Verification items for the finished model (mm, model axes). Round coordinates to 2 decimals unless told otherwise and drop trailing zeros. Write each loop counter-clockwise with the first axis right and the second up, starting at its lowest first coordinate (ties: lowest second). Pieces come first, ordered by that corner, then holes. Notation, with made-up numbers: (-21, -2.75) -> (4, -2.75) arc R17 ccw to (4, 15.25) -> close; hole circle Ø5 at (-1.75, -4). An arc over 180 degrees is marked (long way). Answer as a JSON object with one key per item and string values. Group by question number.
(1) Scan lines: L1, parallel to Y at x = 0, z = 1.7; L2, parallel to Y at x = 123, z = 3.9; L3, parallel to Y at x = 27, z = 0.3. Record each from-to range of solid material in increasing order. Write a range as from..to.
(2) Draft check along X on faces 1 (the face through (5.76, 1, 2.46)), 2 (the face through (189.98, -5.06, 2.46)), 3 (the face through (-4.357, 0, 2)), 4 (the face through (101, 10, 5)). Enter one of: released by +X, released by -X, zero draft, split by the parting line, or undercut.
(3) Gauge pin test, flat ends, axial feed: pin 1 Ø1 at (x, z) = (144.5, 3.5) entering from +Y; pin 2 Ø1 at (y, z) = (3, 0.5) entering from -X; pin 3 Ø1 at (y, z) = (-3, 1) entering from +X. Record the tip position at first contact, or that the pin passes through.
(4) Sectioned sample at C-C on x = 84.5. Record the cut outline in (y, z).
(5) Sectioned sample at B-B on z = 3.2. Record the cut outline in (x, y), and give its area (3 significant figures).
```python
from build123d import *

# Parameters (mm, degrees)
SZKIC1_R                    = 3.000000079
DODANIE_WYCI_GNI_CIE1_DEPTH = 5
SZKIC2_W                    = 1.618528634
SZKIC2_H                    = 7.505645785
SZKIC2_W_2                  = 0.651830256
SZKIC2_H_2                  = 5.051684483
WYTNIJ_WYCI_GNI_CIE3_DEPTH  = 6


with BuildPart() as part:
    # Szkic1 → Dodanie-wyciągnięcie1 (new body)
    with BuildSketch(Plane.XY):
        with BuildLine():
            ThreePointArc((186.046385231, -5.249250637), (192.755682752, 2.359335985), (182.617563383, 2.007484775))
            ThreePointArc((182.617563383, 2.007484775), (181.515861501, 0.778055334), (179.877474491, 0.575739249))
            ThreePointArc((179.877474491, 0.575739249), (94.00112496, 10.812901668), (8.093987839, 0.837396921))
            ThreePointArc((8.093987839, 0.837396921), (5.72392167, 1.013694647), (3.88824622, 2.523194623))
            ThreePointArc((3.88824622, 2.523194623), (-4.363457527, 1.563716145), (1.400567067, -4.418527092))
            ThreePointArc((1.400567067, -4.418527092), (93.788687704, 9.660753619), (186.046385231, -5.249250637))
        make_face()
        Circle(SZKIC1_R, mode=Mode.SUBTRACT)
        with Locations((187.7624, 0)):
            Circle(SZKIC1_R, mode=Mode.SUBTRACT)
    extrude(amount=DODANIE_WYCI_GNI_CIE1_DEPTH)

    # Szkic2 → Wytnij-wyciągnięcie3 (cut, through all)
    with BuildSketch(Plane.XY):
        with Locations((193.638606269, 0.381285041)):
            Rectangle(SZKIC2_W, SZKIC2_H)
        with Locations((-4.682734605, -0.038745932)):
            Rectangle(SZKIC2_W_2, SZKIC2_H_2)
    extrude(amount=WYTNIJ_WYCI_GNI_CIE3_DEPTH, mode=Mode.SUBTRACT)


solid = part.part
```
Computed values:
{
 "1": {"L1": "-4.64..-3, 3..4.64", "L2": "8.11..9.63", "L3": "2.47..4.8"},
 "2": {"face 1": "undercut", "face 2": "split by the parting line", "face 3": "released by -X", "face 4": "zero draft"},
 "3": {"pin 1": "y = 7.34", "pin 2": "x = -3.9", "pin 3": "x = 192.69"},
 "4": {"outline": "(9.56, 0) -> (10.71, 0) -> (10.71, 5) -> (9.56, 5) -> close"},
 "5": {"outline": "(-4.36, -1.58) arc R4.64 ccw to (1.4, -4.42) arc R301.27 cw to (186.05, -5.25) arc R5.52 ccw to (192.83, -2.2) -> (192.83, 2.2) arc R5.52 ccw to (182.62, 2.01) arc R2.35 cw to (179.88, 0.58) arc R370.04 ccw to (8.09, 0.84) arc R3.93 cw to (3.89, 2.52) arc R4.64 ccw to (-4.36, 1.58) -> close; hole circle Ø6 at (0, 0); hole circle Ø6 at (187.76, 0)", "area": "467 mm2"}
}
